Geometry: final body of the model. Coordinates: model frame, mm. A direction names the side the tool comes from. Coordinates: 2 decimals unless noted, no trailing zeros. Order: outer loops, then holes, each group sorted by start corner. A loop starts at its lowest first (then second) coordinate and runs counter-clockwise, first axis right, second up. Notation, with made-up numbers: (-6, -22) -> (48, -22) arc R29 ccw to (48, 4) -> close; hole circle Ø9 at (36.5, 85). An arc over 180 degrees is marked (long way). Answer in a Markdown table with one row per item. Add a question column.
1) Section query A-A on z = 0. Return the cut outline in (x, y) (3 decimals).
2) Section query B-B on x = 0. Return the cut outline in (y, z).
3) Set-up query: faces 1 (the face through (4, -7, -2)), 2 (the face through (0, 11, 0)), 3 (the face through (-3, -16, 1)). Return all of +Z, -Z, +X, -X, +Y, -Y with unobstructed straight access to the full face (end or side cutting, diameter ignored); none if empty.
4) Section query D-D on y = 8. Return the cut outline in (x, z) (3 decimals).
5) Contact query for flat-ended pins moving along their axis: P1, Ø1.8, axis at x = 1.5, z = 0, coming from the -Y side; P2, Ø1.5, axis at y = 4, z = 1, coming from the -X side; P3, Ø1.6, axis at x = 1.75, z = 0, coming from the +Y side. Output: stop coordinate, or through.
6) Pull-direction query (X, two-part tool) for faces 4 (the face through (0, -1, 0)), 5 (the face through (-4, 15, 0)), 6 (the face through (1.457, -3.451, 4.626)); classes: +X half, -X half, draft (parallel to the pull), parting line (faces both ways), or undercut.
7) Section query C-C on x = 1.75. Return the cut outline in (y, z) (3 decimals).
8) Ray query, line 1 (Y direction, x = 1.25, z = 1.75); line 2 (X direction, y = 8.5, z = -0.5) (3 decimals); line 3 (Z direction, x = 1.75, y = 8.25) (3 decimals). Return the intervals inside material, ascending. Write a range as from..to.
```python
from build123d import *

# Parameters (mm, degrees)
SKETCH1_R                          = 4.5
BOSS_EXTRUDE1_DEPTH                = 15
F_6_0MM_DOWEL_HOLE1_D              = 7
F_6_0MM_DOWEL_HOLE1_DEPTH          = 4
SKETCH5_R                          = 4.85
BOSS_EXTRUDE2_DEPTH                = 7
SKETCH6_R                          = 4
BOSS_EXTRUDE3_DEPTH                = 9
F_6_0MM_DOWEL_HOLE2_D              = 6
F_6_0MM_DOWEL_HOLE2_DEPTH          = 15
TAP_DRILL_FOR_M1_6X0_35_TAP3_D     = 1.25
TAP_DRILL_FOR_M1_6X0_35_TAP3_DEPTH = 41


with BuildPart() as part:
    # Sketch1 → Boss-Extrude1 (new body)
    with BuildSketch(Plane(origin=(0, 0, 0), x_dir=(1, 0, 0), z_dir=(0, 1, 0))):
        with Locations(Location((0, 0, 0), (0, 0, 270))):
            Circle(SKETCH1_R)
    extrude(amount=BOSS_EXTRUDE1_DEPTH)

    # Ø6.0mm Dowel Hole1
    with Locations(Plane(origin=(0, 15, 0), x_dir=(1, 0, 0), z_dir=(0, 1, 0))):
        with Locations((0, 0)):
            Hole(F_6_0MM_DOWEL_HOLE1_D / 2, depth=F_6_0MM_DOWEL_HOLE1_DEPTH)

    # Sketch5 → Boss-Extrude2 (add)
    with BuildSketch(Plane(origin=(0, 0, 0), x_dir=(1, 0, 0), z_dir=(0, 1, 0))):
        with Locations(Location((0, 0, 0), (0, 0, 270))):
            Circle(SKETCH5_R)
    extrude(amount=-BOSS_EXTRUDE2_DEPTH)

    # Sketch6 → Boss-Extrude3 (add)
    with BuildSketch(Plane.XZ.offset(7)):
        with Locations(Location((0, 0, 0), (0, 0, 90))):
            Circle(SKETCH6_R)
    extrude(amount=BOSS_EXTRUDE3_DEPTH)

    # Ø6.0mm Dowel Hole2
    with Locations(Plane(origin=(0, -16, 0), x_dir=(-1, 0, 0), z_dir=(0, -1, 0))):
        with Locations((0, 0)):
            Hole(F_6_0MM_DOWEL_HOLE2_D / 2, depth=F_6_0MM_DOWEL_HOLE2_DEPTH)

    # Tap Drill for M1.6x0.35 Tap3
    with Locations(Plane(origin=(0, -1, 0), x_dir=(-1, 0, 0), z_dir=(0, -1, 0))):
        with Locations((1.75, 0), (-1.75, 0)):
            Hole(TAP_DRILL_FOR_M1_6X0_35_TAP3_D / 2, depth=TAP_DRILL_FOR_M1_6X0_35_TAP3_DEPTH)


solid = part.part
```
Result:
| question | item | result |
|---|---|---|
| 1 | outline | (-4.85, -7) -> (-4, -7) -> (-4, -16) -> (-3, -16) -> (-3, -1) -> (-2.375, -1) -> (-2.375, 11) -> (-3.5, 11) -> (-3.5, 15) -> (-4.5, 15) -> (-4.5, 0) -> (-4.85, 0) -> close; (-1.125, -1) -> (1.125, -1) -> (1.125, 11) -> (-1.125, 11) -> close; (2.375, -1) -> (3, -1) -> (3, -16) -> (4, -16) -> (4, -7) -> (4.85, -7) -> (4.85, 0) -> (4.5, 0) -> (4.5, 15) -> (3.5, 15) -> (3.5, 11) -> (2.375, 11) -> close |
| 2 | outline | (-16, -4) -> (-7, -4) -> (-7, -4.85) -> (0, -4.85) -> (0, -4.5) -> (15, -4.5) -> (15, -3.5) -> (11, -3.5) -> (11, 3.5) -> (15, 3.5) -> (15, 4.5) -> (0, 4.5) -> (0, 4.85) -> (-7, 4.85) -> (-7, 4) -> (-16, 4) -> (-16, 3) -> (-1, 3) -> (-1, -3) -> (-16, -3) -> close |
| 3 | face 1 | -Y |
| 3 | face 2 | +Y |
| 3 | face 3 | +Z, -Z, +X, -X, -Y |
| 4 | outline | circle Ø9 at (0, 0); hole circle Ø1.25 at (-1.75, 0); hole circle Ø1.25 at (1.75, 0) |
| 5 | P1 | y = -1 |
| 5 | P2 | x = -4.49 |
| 5 | P3 | y = 11 |
| 6 | face 4 | undercut |
| 6 | face 5 | draft |
| 6 | face 6 | parting line |
| 7 | outline | (-16, -3.597) -> (-7, -3.597) -> (-7, -4.523) -> (0, -4.523) -> (0, -4.146) -> (15, -4.146) -> (15, -3.031) -> (11, -3.031) -> (11, -0.625) -> (-1, -0.625) -> (-1, -2.437) -> (-16, -2.437) -> close; (-16, 2.437) -> (-1, 2.437) -> (-1, 0.625) -> (11, 0.625) -> (11, 3.031) -> (15, 3.031) -> (15, 4.146) -> (0, 4.146) -> (0, 4.523) -> (-7, 4.523) -> (-7, 3.597) -> (-16, 3.597) -> close |
| 8 | line 1 | -1..11 |
| 8 | line 2 | -4.472..-2.125, -1.375..1.375, 2.125..4.472 |
| 8 | line 3 | -4.146..-0.625, 0.625..4.146 |
